Model file for the job. Use its own axes, mm. Face numbers are marked on the shaded views. A direction names the side the tool comes from. Coordinates: 2 decimals unless noted, no trailing zeros. Loops run counter-clockwise (first coordinate to the right, second up) from the corner with the lowest first, then second, coordinate; pieces in that order, holes last.
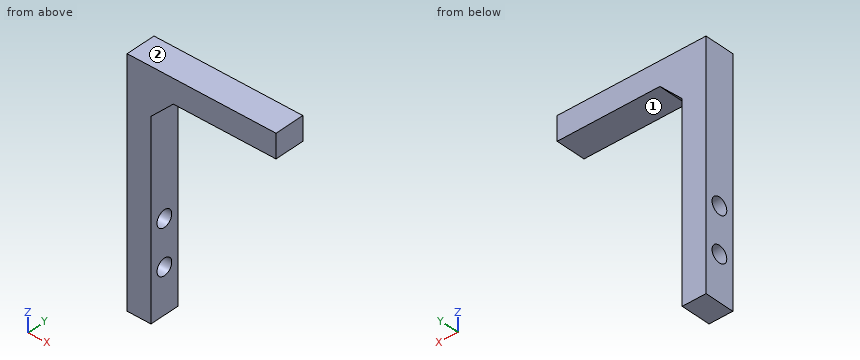
from build123d import *

# Parameters (mm, degrees)
EXTRUDE_1_DEPTH     = 10
CHAMFER_1_SIZE      = 7.5
SKETCH_2_R          = 2.75
CUT_EXTRUDE_1_DEPTH = 80.959868111


with BuildPart() as part:
    # 草图1 → 凸台-拉伸1 (new body)
    with BuildSketch(Plane(origin=(0, 0, 0), x_dir=(1, 0, 0), z_dir=(0, 1, 0))):
        Polygon((-10.992805755, 67.302158273), (-18.992805755, 67.302158273), (-18.992805755, -4.697841727), (-18.992805755, -12.697841727), (-10.992805755, -12.697841727), (31.007194245, -12.697841727), (31.007194245, -4.697841727), (-10.992805755, -4.697841727), align=None)
    extrude(amount=EXTRUDE_1_DEPTH)

    # 倒角1
    chamfer_1_edges = [part.edges().sort_by_distance(p)[0] for p in [
        (-10.992805755, 5, 4.697841727),
    ]]
    chamfer(chamfer_1_edges, length=CHAMFER_1_SIZE)

    # 草图2 → 切除-拉伸1 (cut, through all)
    with BuildSketch(Plane(origin=(-10.992805755, 0, 0), x_dir=(0, 0, -1), z_dir=(1, 0, 0))):
        with Locations((37.302158273, 5)):
            Circle(SKETCH_2_R)
        with Locations((52.302158273, 5)):
            Circle(SKETCH_2_R)
    extrude(amount=-CUT_EXTRUDE_1_DEPTH, mode=Mode.SUBTRACT)


solid = part.part
Q1. Slice it at C-C (z = -51.5). List the corners of the cut face in (x, y), and give its area (3 significant figures).
Answers:
outline: (-18.99, 0) - (-10.99, 0) - (-10.99, 2.37) - (-18.99, 2.37) - close; (-18.99, 7.63) - (-10.99, 7.63) - (-10.99, 10) - (-18.99, 10) - close
area: 37.9 mm2
Q2. Slice it at B-B (y = 1). List the corners of the cut face in (x, z), and give its area (3 significant figures).
Answers:
outline: (-18.99, -67.3) - (-10.99, -67.3) - (-10.99, -2.8) - (-3.49, 4.7) - (31.01, 4.7) - (31.01, 12.7) - (-18.99, 12.7) - close
area: 1,000 mm2
Q3. Which spindle directions (+Z, -Z, +X, -X, +Y, -Y) get a long thin tool onto all of the face, cutting with end or side? Do the marked faces 1 and 2. Say none if no direction does.
Answers:
face 1: -Z, +X, +Y, -Y
face 2: +Z, +X, -X, +Y, -Y
Q4. Drill centre lines: line 1 (Z direction, x = 16, y = 3.75); line 2 (Z direction, x = -12, y = 5.75); line 3 (X direction, y = 7.75, z = -57). Where is each one in solid material? Low to high.
Answers:
line 1: z = 4.7 to 12.7
line 2: z = -67.3 to -54.95, -49.66 to -39.95, -34.66 to 12.7
line 3: x = -18.99 to -10.99
Q5. Slice it at A-A (y = 5). List the corners of the cut face in (x, z), and give its area (3 significant figures).
Answers:
outline: (-18.99, -67.3) - (-10.99, -67.3) - (-10.99, -55.05) - (-18.99, -55.05) - close; (-18.99, -49.55) - (-10.99, -49.55) - (-10.99, -40.05) - (-18.99, -40.05) - close; (-18.99, -34.55) - (-10.99, -34.55) - (-10.99, -2.8) - (-3.49, 4.7) - (31.01, 4.7) - (31.01, 12.7) - (-18.99, 12.7) - close
area: 916 mm2
Q6. Flat gauge pins, fed straight in: P1, Ø3, axis at y = 5.5, z = -21, coming from the +X side; P2, Ø5, axis at x = 11, y = 2.5, coming from the -Z side. Where does each tip first touch, or does it go through?
Answers:
P1: stops at x = -10.99
P2: stops at z = 4.7
Q7. Slice it at D-D (x = 2.5). List the corners of the cut face in (y, z), and give its area (3 significant figures).
Answers:
outline: (0, 4.7) - (10, 4.7) - (10, 12.7) - (0, 12.7) - close
area: 80.0 mm2
